Drawing for the job (mm, zero at the part's lowest x, y, z). A direction names the side the tool comes from. Give positions to 0.01 mm unless a question says otherwise; leave off trailing zeros. Write each loop counter-clockwise with the first axis right and the second up, starting at its lowest first coordinate (ties: lowest second). Pieces come first, ordered by that corner, then holes. Notation, with made-up numbers: M 7.25,-21.75 L 64.25,-21.75 A14 ccw 64.25,-9.75 Z; hole C 26,70.25 d8. An arc over 180 degrees is marked long. Answer as a JSON object with one key per item and string values. Group by question number.
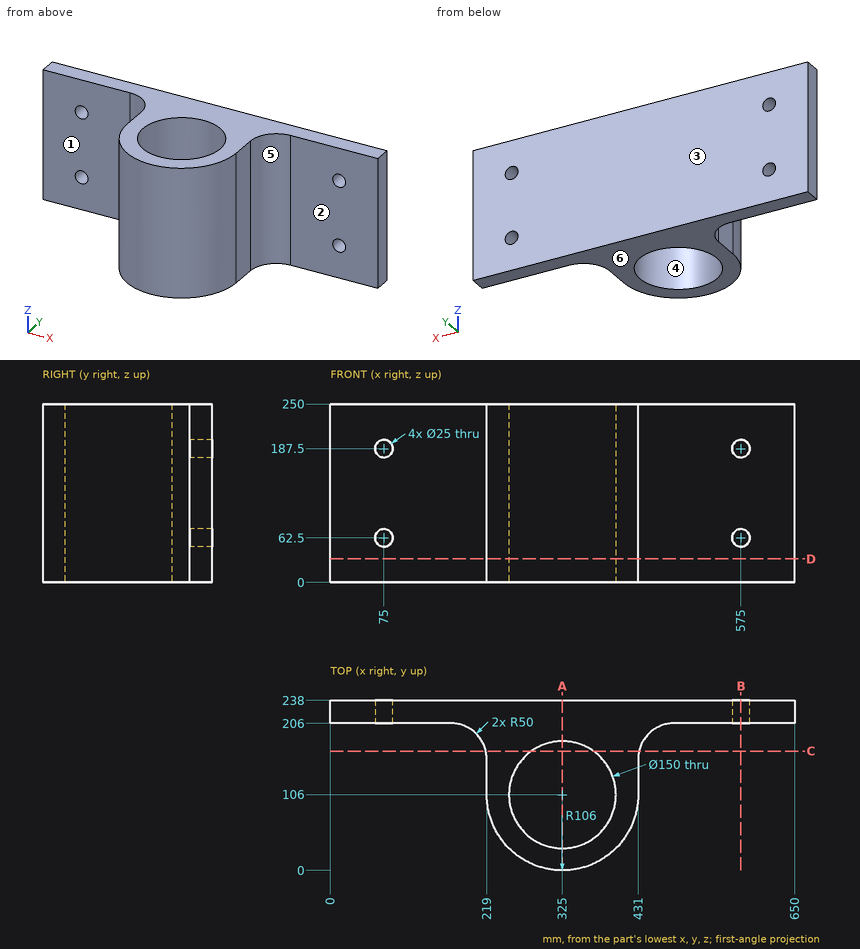
Q1. Slice it at B-B, the plane x = 575. Write the cut outline in (y, z), then the cut area to 3 significant figures.
Q2. Slice it at A-A, the plane x = 325. Write the cut outline in (y, z).
Q3. Drop flat-ended pins along their axis: P1, Ø2, axis at y = 130, z = 194, coming from the +X side; P2, Ø1.5, axis at y = 30, z = 69, coming from the -X side; P3, Ø1.5, axis at y = 112, z = 196, coming from the -X side; P4, Ø22.5, axis at x = 575, z = 187.5, coming from the -Y side (1 decimal). Give the stop position or say it passes through.
Q4. 3-axis set-ups, long thin cutter, end or side, ignore diameter. For the marked faces 1, 2 and 3: which of +Z, -Z, +X, -X, +Y, -Y reach the whole face in a straight line?
Q5. Slice it at C-C, the plane y = 167. Write the cut outline in (x, z) (3 decimals).
Q6. Wall check: L1, parallel to X at y = 215, z = 62.5; L2, parallel to Z at x = 75, y = 223; L3, parallel to Y at x = 325, z = 179. Give the ranges that are in metal, low to high.
Q7. Two-plate mould, pull along X, no slides. Class the marked faces 4, 5 and 6: +X half, -X half, draft (parallel to the pull), parting line (faces both ways), or undercut.
Q8. Slice it at D-D, the plane z = 33. Write the cut outline in (x, y), then the cut area to 3 significant figures.
Solved:
{
 "1": {"outline": "M 206,0 L 238,0 L 238,50 L 206,50 Z; M 206,75 L 238,75 L 238,175 L 206,175 Z; M 206,200 L 238,200 L 238,250 L 206,250 Z", "area": "6,400 mm²"},
 "2": {"outline": "M 0,0 L 31,0 L 31,250 L 0,250 Z; M 181,0 L 238,0 L 238,250 L 181,250 Z"},
 "3": {"P1": "stops at x = 431", "P2": "stops at x = 250.34", "P3": "stops at x = 219", "P4": "passes through"},
 "4": {"face 1": "+Z, -Z, -X, -Y", "face 2": "+Z, -Z, +X, -Y", "face 3": "+Z, -Z, +X, -X, +Y"},
 "5": {"outline": "M 217.775,0 L 281.365,0 L 281.365,250 L 217.775,250 Z; M 368.635,0 L 432.225,0 L 432.225,250 L 368.635,250 Z"},
 "6": {"L1": "x = 0 to 62.5, 87.5 to 562.5, 587.5 to 650", "L2": "z = 0 to 50, 75 to 175, 200 to 250", "L3": "y = 0 to 31, 181 to 238"},
 "7": {"face 4": "undercut", "face 5": "+X half", "face 6": "draft"},
 "8": {"outline": "M 0,206 L 169,206 A50 cw 219,156 L 219,106 A106 ccw 431,106 L 431,156 A50 cw 481,206 L 650,206 L 650,238 L 0,238 Z; hole C 325,106 d150", "area": "43,100 mm²"}
}
